Model file for the job. Use its own axes, mm. A direction names the side the tool comes from. Round coordinates to 2 decimals unless told otherwise and drop trailing zeros. Loops run counter-clockwise (first coordinate to the right, second up) from the corner with the lowest first, then second, coordinate; pieces in that order, holes last.
Autodesk Inventor part; units mm, degrees
ref_plane "YZ Plane" through (0, 0, 0) normal (1, 0, 0) x (0, 1, 0)
ref_plane "XZ Plane" through (0, 0, 0) normal (0, 1, 0) x (-1, 0, 0)
ref_plane "XY Plane" through (0, 0, 0) normal (0, 0, 1) x (1, 0, 0)
sketch "Sketch1" plane through (0, 0, 0) normal (0, 1, 0) x (-1, 0, 0)
  line L0 (0, 0) -> (0, 13)
  line L1 (-8.9, 13) -> (-7.9, 11.5)
  line L2 (-7.9, 11.5) -> (-7.9, 5.6)
  line L3 (-7.9, 5.6) -> (-8.5, 5)
  line L4 (-8.5, 5) -> (-8.5, 0)
  line L5 (-8.5, 0) -> (-9.5, 0)
  line L6 (-9.5, 0) -> (-9.5, 13)
  line L7 (-9.5, 13) -> (-8.9, 13)
  line L8 (-9.5, 0.8) -> (-9.9, 0.4)
  line L9 (-9.9, 0.4) -> (-9.9, 0)
  line L10 (-9.9, 0) -> (-9.5, 0)
  dimension "d0" = 15.8
  dimension "d1" = 5
  dimension "d2" = 19
  dimension "d3" = 1
  dimension "d4" = 1.5
  dimension "d5" = 8
  dimension "d6" = 17
  dimension "d7" = 45
  dimension "d9" = 0.8
  dimension "d10" = 0.4
  dimension "d11" = 0.4
revolve "Revolution1" add sketch "Sketch1" angle 360 about axis through (0, 0, 0) along (0, 0, 1)
ref_plane "Work Plane1" through (0, 0, 2.5) normal (0, 0, -1) x (-1, 0, 0)
sketch "Sketch2" plane through (0, 0, 2.5) normal (0, 0, -1) x (-1, 0, 0)
  circle A0 centre (0, 0) radius 8.5
  line L0 (-2.2, 8.2104) -> (-2.2, 7.6916)
  arc A1 (-2.2, 7.6916) -> (-7.6916, 2.2) centre (0, 0) ccw
  line L1 (-7.6916, 2.2) -> (-8.2104, 2.2)
  dimension "d14" = 60
  dimension "d15" = 0.5
extrude "Extrusion1" add sketch "Sketch2" along normal mid plane 3 contours L0 A1 L1 A0 picked at (-5.6701, 6.0517)
chamfer "Chamfer1" distance 0.5 angle 45 2 edges at (5.6569, 5.6569, 4) (5.6569, 5.6569, 1)
pattern_circular "Circular Pattern1" count 4 over 360 about axis through (0, 0, -10) along (0, 0, 1) of "Extrusion1", "Chamfer1"
properties part number "screw-grip_3DPrint"
Q1. Slice it at A-A on x = 0. Give the cut face in (y, z).
Q2. Flat gauge pins, fed straight in: P1, Ø0.6, axis at y = 8, z = 3, coming from the +X side; P2, Ø1.5, axis at x = -1.5, y = 6.5, coming from the +Z side; P3, Ø1.8, axis at x = 5, y = 6, coming from the +Z side; P4, Ø6, axis at x = 6, z = 4.5, coming from the -Y side. Where does each tip first touch, or does it go through?
Q3. Slice it at C-C on z = 2.25. Give the cut face in (x, y).
Q4. Tool access for faces 4 (the face through (-8.49, -0.37, 2.46)), 5 (the face through (-6.269, 4.807, 8.509)), 6 (the face through (-5.697, -5.617, 2.514)): list every direction of +Z, -Z, +X, -X, +Y, -Y with a clear straight run to the whole face (end or side of a thin tool).
Q5. Pull direction Z, two halves, no side cores. Call faces 1 (the face through (5.8, 5.715, 3.643)), 2 (the face through (-5.715, -5.8, 1.357)), 3 (the face through (4.38, -8.43, 6.99)): pulls with the +Z half, pulls with the -Z half, needs draft (parallel to the pull), parting line crosses it, or undercut.
Q6. Probe line 1 (Y direction, x = 0, z = 1.6); line 2 (Y direction, x = 0, z = 7.75); line 3 (X direction, y = 1, z = 9.5). List the from-to ranges inside material, lowest first.
Q7. Slice it at D-D on z = 10.25. Give the cut face in (x, y), plus the area to 3 significant figures.
Reply:
1. outline: (-9.9, 0) - (-8.5, 0) - (-8.5, 5) - (-7.9, 5.6) - (-7.9, 11.5) - (-8.9, 13) - (-9.5, 13) - (-9.5, 0.8) - (-9.9, 0.4) - close; (7.9, 5.6) - (8.5, 5) - (8.5, 0) - (9.9, 0) - (9.9, 0.4) - (9.5, 0.8) - (9.5, 13) - (8.9, 13) - (7.9, 11.5) - close
2. P1: stops at x = 5.56
2. P2: passes through
2. P3: stops at z = 12.72
2. P4: stops at y = -9.01
3. outline: circle Ø19 at (0, 0); hole (-8.21, -2.2) - (-7.69, -2.2) arc R8 ccw to (-2.2, -7.69) - (-2.2, -8.21) arc R8.5 ccw to (2.2, -8.21) - (2.2, -7.69) arc R8 ccw to (7.69, -2.2) - (8.21, -2.2) arc R8.5 ccw to (8.21, 2.2) - (7.69, 2.2) arc R8 ccw to (2.2, 7.69) - (2.2, 8.21) arc R8.5 ccw to (-2.2, 8.21) - (-2.2, 7.69) arc R8 ccw to (-7.69, 2.2) - (-8.21, 2.2) arc R8.5 ccw to start
4. face 4: none
4. face 5: +Z, -Z
4. face 6: -Z
5. face 1: undercut
5. face 2: pulls with the -Z half
5. face 3: needs draft
6. line 1: y = -9.5 to -8.5, 8.5 to 9.5
6. line 2: y = -9.5 to -7.9, 7.9 to 9.5
6. line 3: x = -9.45 to -7.84, 7.84 to 9.45
7. outline: circle Ø19 at (0, 0); hole circle Ø15.8 at (0, 0)
7. area: 87.5 mm2
